```python
from build123d import *

# Parameters (mm, degrees)
F0_R     = 22.5
F1_DEPTH = 7.5
F2_R     = 2
F3_DEPTH = 5
F4_DEPTH = 5
F5_R     = 22.5
F5_R_2   = 10
F6_DEPTH = 1.5


with BuildPart() as f1:
    # F0 (on Top) → F1 (new body)
    with BuildSketch(Plane.XY):
        Circle(F0_R)
        with BuildLine():
            ThreePointArc((15.973986, 0.912023), (15.993495, 0.456197), (16, 0))
            ThreePointArc((16, 0), (15.925079, -1.546568), (15.701016, -3.078652))
            ThreePointArc((15.701016, -3.078652), (15.665345, -3.255296), (15.627688, -3.431527))
            ThreePointArc((15.627688, -3.431527), (15.076175, -5.358074), (14.288169, -7.200571))
            ThreePointArc((14.288169, -7.200571), (14.206163, -7.361041), (14.122356, -7.520577))
            ThreePointArc((14.122356, -7.520577), (13.071518, -9.226885), (11.815634, -10.788456))
            ThreePointArc((11.815634, -10.788456), (11.693375, -10.92085), (11.569633, -11.051859))
            ThreePointArc((11.569633, -11.051859), (10.097407, -12.411381), (8.466788, -13.576211))
            ThreePointArc((8.466788, -13.576211), (8.313343, -13.67071), (8.158844, -13.763476))
            ThreePointArc((8.158844, -13.763476), (6.374417, -14.675381), (4.489999, -15.35708))
            ThreePointArc((4.489999, -15.35708), (4.316748, -15.406677), (4.14295, -15.454319))
            ThreePointArc((4.14295, -15.454319), (2.178666, -15.850975), (0.180207, -15.998985))
            ThreePointArc((0.180207, -15.998985), (0, -16), (-0.180207, -15.998985))
            ThreePointArc((-0.180207, -15.998985), (-2.178666, -15.850975), (-4.14295, -15.454319))
            ThreePointArc((-4.14295, -15.454319), (-4.316748, -15.406677), (-4.489999, -15.35708))
            ThreePointArc((-4.489999, -15.35708), (-6.374417, -14.675381), (-8.158844, -13.763476))
            ThreePointArc((-8.158844, -13.763476), (-8.313343, -13.67071), (-8.466788, -13.576211))
            ThreePointArc((-8.466788, -13.576211), (-10.097407, -12.411381), (-11.569633, -11.051859))
            ThreePointArc((-11.569633, -11.051859), (-11.693375, -10.92085), (-11.815634, -10.788456))
            ThreePointArc((-11.815634, -10.788456), (-13.071518, -9.226885), (-14.122356, -7.520577))
            ThreePointArc((-14.122356, -7.520577), (-14.206163, -7.361041), (-14.288169, -7.200571))
            ThreePointArc((-14.288169, -7.200571), (-15.076175, -5.358074), (-15.627688, -3.431527))
            ThreePointArc((-15.627688, -3.431527), (-15.665345, -3.255296), (-15.701016, -3.078652))
            ThreePointArc((-15.701016, -3.078652), (-15.9627, -1.091879), (-15.973986, 0.912023))
            ThreePointArc((-15.973986, 0.912023), (-15.9627, 1.091879), (-15.94939, 1.271596))
            ThreePointArc((-15.94939, 1.271596), (-15.665345, 3.255296), (-15.135566, 5.187932))
            ThreePointArc((-15.135566, 5.187932), (-15.076175, 5.358074), (-15.014871, 5.527536))
            ThreePointArc((-15.014871, 5.527536), (-14.206163, 7.361041), (-13.174611, 9.079076))
            ThreePointArc((-13.174611, 9.079076), (-13.071518, 9.226885), (-12.966768, 9.373523))
            ThreePointArc((-12.966768, 9.373523), (-11.693375, 10.92085), (-10.236555, 12.296867))
            ThreePointArc((-10.236555, 12.296867), (-10.097407, 12.411381), (-9.956978, 12.52432))
            ThreePointArc((-9.956978, 12.52432), (-8.313343, 13.67071), (-6.539301, 14.602655))
            ThreePointArc((-6.539301, 14.602655), (-6.374417, 14.675381), (-6.208726, 14.746245))
            ThreePointArc((-6.208726, 14.746245), (-4.316748, 15.406677), (-2.357056, 15.825432))
            ThreePointArc((-2.357056, 15.825432), (-2.178666, 15.850975), (-2, 15.874508))
            ThreePointArc((-2, 15.874508), (0, 16), (2, 15.874508))
            ThreePointArc((2, 15.874508), (2.178666, 15.850975), (2.357056, 15.825432))
            ThreePointArc((2.357056, 15.825432), (4.316748, 15.406677), (6.208726, 14.746245))
            ThreePointArc((6.208726, 14.746245), (6.374417, 14.675381), (6.539301, 14.602655))
            ThreePointArc((6.539301, 14.602655), (8.313343, 13.67071), (9.956978, 12.52432))
            ThreePointArc((9.956978, 12.52432), (10.097407, 12.411381), (10.236555, 12.296867))
            ThreePointArc((10.236555, 12.296867), (11.693375, 10.92085), (12.966768, 9.373523))
            ThreePointArc((12.966768, 9.373523), (13.071518, 9.226885), (13.174611, 9.079076))
            ThreePointArc((13.174611, 9.079076), (14.206163, 7.361041), (15.014871, 5.527536))
            ThreePointArc((15.014871, 5.527536), (15.076175, 5.358074), (15.135566, 5.187932))
            ThreePointArc((15.135566, 5.187932), (15.665345, 3.255296), (15.94939, 1.271596))
            ThreePointArc((15.94939, 1.271596), (15.9627, 1.091879), (15.973986, 0.912023))
        make_face(mode=Mode.SUBTRACT)
        with BuildLine():
            ThreePointArc((0, 14), (1.22661, 14.695473), (2, 15.874508))
            ThreePointArc((2, 15.874508), (0, 16), (-2, 15.874508))
            ThreePointArc((-2, 15.874508), (-1.22661, 14.695473), (0, 14))
        make_face()
        with BuildLine():
            ThreePointArc((-3.777155, 13.480842), (-2.783667, 14.481461), (-2.357056, 15.825432))
            ThreePointArc((-2.357056, 15.825432), (-4.316748, 15.406677), (-6.208726, 14.746245))
            ThreePointArc((-6.208726, 14.746245), (-5.145915, 13.81959), (-3.777155, 13.480842))
        make_face()
        with BuildLine():
            ThreePointArc((-7.274175, 11.961872), (-6.587493, 13.193424), (-6.539301, 14.602655))
            ThreePointArc((-6.539301, 14.602655), (-8.313343, 13.67071), (-9.956978, 12.52432))
            ThreePointArc((-9.956978, 12.52432), (-8.683571, 11.918771), (-7.274175, 11.961872))
        make_face()
        with BuildLine():
            ThreePointArc((-10.231703, 9.555744), (-9.902754, 10.926892), (-10.236555, 12.296867))
            ThreePointArc((-10.236555, 12.296867), (-11.693375, 10.92085), (-12.966768, 9.373523))
            ThreePointArc((-12.966768, 9.373523), (-11.577207, 9.133991), (-10.231703, 9.555744))
        make_face()
        with BuildLine():
            ThreePointArc((-12.430393, 6.440911), (-12.483573, 7.849962), (-13.174611, 9.079076))
            ThreePointArc((-13.174611, 9.079076), (-14.206163, 7.361041), (-15.014871, 5.527536))
            ThreePointArc((-15.014871, 5.527536), (-13.612214, 5.671785), (-12.430393, 6.440911))
        make_face()
        with BuildLine():
            ThreePointArc((-13.707177, 2.848384), (-14.138543, 4.190837), (-15.135566, 5.187932))
            ThreePointArc((-15.135566, 5.187932), (-15.665345, 3.255296), (-15.94939, 1.271596))
            ThreePointArc((-15.94939, 1.271596), (-14.637665, 1.788928), (-13.707177, 2.848384))
        make_face()
        with BuildLine():
            ThreePointArc((-15.973986, 0.912023), (-15.9627, -1.091879), (-15.701016, -3.078652))
            ThreePointArc((-15.701016, -3.078652), (-14.577508, -2.226605), (-13.967363, -0.955394))
            ThreePointArc((-13.967363, -0.955394), (-14.744922, 0.220896), (-15.973986, 0.912023))
        make_face()
        with BuildLine():
            ThreePointArc((-15.627688, -3.431527), (-15.076175, -5.358074), (-14.288169, -7.200571))
            ThreePointArc((-14.288169, -7.200571), (-13.436204, -6.077001), (-13.191653, -4.688315))
            ThreePointArc((-13.191653, -4.688315), (-14.257737, -3.765428), (-15.627688, -3.431527))
        make_face()
        with BuildLine():
            ThreePointArc((-14.122356, -7.520577), (-13.071518, -9.226885), (-11.815634, -10.788456))
            ThreePointArc((-11.815634, -10.788456), (-11.298397, -9.476694), (-11.437579, -8.073525))
            ThreePointArc((-11.437579, -8.073525), (-12.713121, -7.472487), (-14.122356, -7.520577))
        make_face()
        with BuildLine():
            ThreePointArc((-11.569633, -11.051859), (-10.097407, -12.411381), (-8.466788, -13.576211))
            ThreePointArc((-8.466788, -13.576211), (-8.322641, -12.173543), (-8.835231, -10.859958))
            ThreePointArc((-8.835231, -10.859958), (-10.225631, -10.625346), (-11.569633, -11.051859))
        make_face()
        with BuildLine():
            ThreePointArc((-8.158844, -13.763476), (-6.374417, -14.675381), (-4.489999, -15.35708))
            ThreePointArc((-4.489999, -15.35708), (-4.729632, -13.967537), (-5.577615, -12.840958))
            ThreePointArc((-5.577615, -12.840958), (-6.979753, -12.990171), (-8.158844, -13.763476))
        make_face()
        with BuildLine():
            ThreePointArc((-4.14295, -15.454319), (-2.178666, -15.850975), (-0.180207, -15.998985))
            ThreePointArc((-0.180207, -15.998985), (-0.785848, -14.725622), (-1.906333, -13.869603))
            ThreePointArc((-1.906333, -13.869603), (-3.216219, -14.391575), (-4.14295, -15.454319))
        make_face()
        with BuildLine():
            ThreePointArc((0.180207, -15.998985), (2.178666, -15.850975), (4.14295, -15.454319))
            ThreePointArc((4.14295, -15.454319), (3.216219, -14.391575), (1.906333, -13.869603))
            ThreePointArc((1.906333, -13.869603), (0.785848, -14.725622), (0.180207, -15.998985))
        make_face()
        with BuildLine():
            ThreePointArc((4.489999, -15.35708), (6.374417, -14.675381), (8.158844, -13.763476))
            ThreePointArc((8.158844, -13.763476), (6.979753, -12.990171), (5.577615, -12.840958))
            ThreePointArc((5.577615, -12.840958), (4.729632, -13.967537), (4.489999, -15.35708))
        make_face()
        with BuildLine():
            ThreePointArc((8.466788, -13.576211), (10.097407, -12.411381), (11.569633, -11.051859))
            ThreePointArc((11.569633, -11.051859), (10.225631, -10.625346), (8.835231, -10.859958))
            ThreePointArc((8.835231, -10.859958), (8.322641, -12.173543), (8.466788, -13.576211))
        make_face()
        with BuildLine():
            ThreePointArc((11.815634, -10.788456), (13.071518, -9.226885), (14.122356, -7.520577))
            ThreePointArc((14.122356, -7.520577), (12.713121, -7.472487), (11.437579, -8.073525))
            ThreePointArc((11.437579, -8.073525), (11.298397, -9.476694), (11.815634, -10.788456))
        make_face()
        with BuildLine():
            ThreePointArc((14.288169, -7.200571), (15.076175, -5.358074), (15.627688, -3.431527))
            ThreePointArc((15.627688, -3.431527), (14.257737, -3.765428), (13.191653, -4.688315))
            ThreePointArc((13.191653, -4.688315), (13.436204, -6.077001), (14.288169, -7.200571))
        make_face()
        with BuildLine():
            ThreePointArc((15.701016, -3.078652), (15.925079, -1.546568), (16, 0))
            ThreePointArc((16, 0), (15.993495, 0.456197), (15.973986, 0.912023))
            ThreePointArc((15.973986, 0.912023), (14.744922, 0.220896), (13.967363, -0.955394))
            ThreePointArc((13.967363, -0.955394), (14.577508, -2.226605), (15.701016, -3.078652))
        make_face()
        with BuildLine():
            ThreePointArc((13.707177, 2.848384), (14.637665, 1.788928), (15.94939, 1.271596))
            ThreePointArc((15.94939, 1.271596), (15.665345, 3.255296), (15.135566, 5.187932))
            ThreePointArc((15.135566, 5.187932), (14.138543, 4.190837), (13.707177, 2.848384))
        make_face()
        with BuildLine():
            ThreePointArc((12.430393, 6.440911), (13.612214, 5.671785), (15.014871, 5.527536))
            ThreePointArc((15.014871, 5.527536), (14.206163, 7.361041), (13.174611, 9.079076))
            ThreePointArc((13.174611, 9.079076), (12.483573, 7.849962), (12.430393, 6.440911))
        make_face()
        with BuildLine():
            ThreePointArc((10.231703, 9.555744), (11.577207, 9.133991), (12.966768, 9.373523))
            ThreePointArc((12.966768, 9.373523), (11.693375, 10.92085), (10.236555, 12.296867))
            ThreePointArc((10.236555, 12.296867), (9.902754, 10.926892), (10.231703, 9.555744))
        make_face()
        with BuildLine():
            ThreePointArc((7.274175, 11.961872), (8.683571, 11.918771), (9.956978, 12.52432))
            ThreePointArc((9.956978, 12.52432), (8.313343, 13.67071), (6.539301, 14.602655))
            ThreePointArc((6.539301, 14.602655), (6.587493, 13.193424), (7.274175, 11.961872))
        make_face()
        with BuildLine():
            ThreePointArc((3.777155, 13.480842), (5.145915, 13.81959), (6.208726, 14.746245))
            ThreePointArc((6.208726, 14.746245), (4.316748, 15.406677), (2.357056, 15.825432))
            ThreePointArc((2.357056, 15.825432), (2.783667, 14.481461), (3.777155, 13.480842))
        make_face()
    extrude(amount=F1_DEPTH)

    # F2 (on face) → F3 (join)
    with BuildSketch(Plane(origin=(0, 0, 0), x_dir=(1, 0, 0), z_dir=(0, 0, -1))):
        with Locations((0, 19)):
            Circle(F2_R)
        with Locations((-19, 0)):
            Circle(F2_R)
        with Locations((19, 0)):
            Circle(F2_R)
        with Locations((0, -19)):
            Circle(F2_R)
    extrude(amount=F3_DEPTH)

    # F2 (on face) → F4 (cut)
    with BuildSketch(Plane(origin=(0, 0, 0), x_dir=(1, 0, 0), z_dir=(0, 0, -1))):
        with Locations((-13.435029, 13.435029)):
            Circle(F2_R)
        with Locations((13.435029, 13.435029)):
            Circle(F2_R)
        with Locations((-13.435029, -13.435029)):
            Circle(F2_R)
        with Locations((13.435029, -13.435029)):
            Circle(F2_R)
    extrude(amount=-F4_DEPTH, mode=Mode.SUBTRACT)

    # F5 (on face) → F6 (join)
    with BuildSketch(Plane.XY.offset(7.5)):
        Circle(F5_R)
        Circle(F5_R_2, mode=Mode.SUBTRACT)
    extrude(amount=F6_DEPTH)


solid = f1.part
```
Geometry: final body of the model. Coordinates: model frame, mm. A direction names the side the tool comes from. Round coordinates to 2 decimals unless told otherwise and drop trailing zeros. Write each loop counter-clockwise with the first axis right and the second up, starting at its lowest first coordinate (ties: lowest second). Pieces come first, ordered by that corner, then holes. Notation, with made-up numbers: (32.5, 77.25) -> (58.5, 77.25) arc R29 ccw to (58.5, 103.25) -> close; hole circle Ø4 at (71, 42.25). An arc over 180 degrees is marked (long way). Return JSON: item names as keys, results as strings.
Q1. Ray query, line 1 (Y direction, x = 2, z = 8); line 2 (X direction, y = 9, z = 4.5); line 3 (Z direction, x = 17, y = 2). Return the intervals inside material, ascending.
From the geometry:
{"line 1": "-22.41 to -9.8, 9.8 to 22.41", "line 2": "-20.62 to -13.1, 13.1 to 20.62", "line 3": "0 to 9"}
Q2. Section D-D on y = -6. Return the cut outline in (x, z), and give its area (3 significant figures).
From the geometry:
{"outline": "(-21.69, 0) -> (-13.4, 0) -> (-13.4, 7.5) -> (-8, 7.5) -> (-8, 9) -> (-21.69, 9) -> close; (8, 7.5) -> (13.4, 7.5) -> (13.4, 0) -> (21.69, 0) -> (21.69, 9) -> (8, 9) -> close", "area": "165 mm2"}
Q3. First-contact query: pin 1 Ø5 at (y, z) = (8.5, 3.5) entering from +X; pin 2 Ø12 at (x, y) = (17.5, -11) entering from -Z; pin 3 Ø1 at (x, z) = (-2.5, 1.5) entering from +Y. Flat tips, straight axial feed; report the tip coordinate or a pass-through.
From the geometry:
{"pin 1": "x = 21.69", "pin 2": "z = 0", "pin 3": "y = 22.41"}
Q4. Section B-B on x = 19. Return the cut outline in (y, z), and give its area (3 significant figures).
From the geometry:
{"outline": "(-12.05, 0) -> (-2, 0) -> (-2, -5) -> (2, -5) -> (2, 0) -> (12.05, 0) -> (12.05, 9) -> (-12.05, 9) -> close", "area": "237 mm2"}
Q5. Mould query, pull axis X, two halves, no side actions, for faces 1 (the cylindrical face through (10.246, -10.627, 3.698)), 2 (the cylindrical face through (10.382, -19.961, 4.437)), 3 (the flat face through (19, 0, -5)). Classes: +X half, -X half, draft (parallel to the pull), parting line (faces both ways), or undercut.
From the geometry:
{"face 1": "undercut", "face 2": "parting line", "face 3": "draft"}
Q6. Section A-A on y = 0. Return the cut outline in (x, z).
From the geometry:
{"outline": "(-22.5, 0) -> (-21, 0) -> (-21, -5) -> (-17, -5) -> (-17, 0) -> (-14.53, 0) -> (-14.53, 7.5) -> (-10, 7.5) -> (-10, 9) -> (-22.5, 9) -> close; (10, 7.5) -> (14.53, 7.5) -> (14.53, 0) -> (17, 0) -> (17, -5) -> (21, -5) -> (21, 0) -> (22.5, 0) -> (22.5, 9) -> (10, 9) -> close"}
Q7. Set-up query: faces 4 (the cylindrical face through (-14.128, 4.174, 3.698)), 5 (the cylindrical face through (-2.17, -9.76, 8.24)). Return all of +Z, -Z, +X, -X, +Y, -Y with unobstructed straight access to the full face (end or side cutting, diameter ignored); none if empty.
From the geometry:
{"face 4": "-Z", "face 5": "+Z, -Z"}
